Geometry check sheet. Reference: the model listing, model coordinates, mm. Face numbers are marked on the shaded views. A direction names the side the tool comes from. Round coordinates to 2 decimals unless told otherwise and drop trailing zeros. Write each loop counter-clockwise with the first axis right and the second up, starting at its lowest first coordinate (ties: lowest second). Pieces come first, ordered by that corner, then holes. Notation, with made-up numbers: (29, -15) -> (50, -15) arc R9 ccw to (50, -1) -> close; hole circle Ø8 at (47.5, 32). An arc over 180 degrees is marked (long way). One line per question, with ' | ' between items.
Autodesk Inventor part; units mm, degrees
ref_plane "YZ Plane" through (0, 0, 0) normal (1, 0, 0) x (0, 1, 0)
ref_plane "XZ Plane" through (0, 0, 0) normal (0, 1, 0) x (-1, 0, 0)
ref_plane "XY Plane" through (0, 0, 0) normal (0, 0, 1) x (1, 0, 0)
sketch "スケッチ1" plane through (0, 0, 0) normal (0, 0, 1) x (1, 0, 0)
  arc A0 (-1.55, 2.6268) -> (1.55, 2.6268) centre (0, 0) ccw
  circle A1 centre (-7, 0) radius 1.6
  circle A2 centre (7, 0) radius 1.6
  arc A3 (-7, 4) -> (-11, 0) centre (-7, 0) ccw
  arc A4 (11, 0) -> (7, 4) centre (7, 0) ccw
  line L0 (-1.55, 10) -> (-1.55, 2.6268)
  line L1 (1.55, 10) -> (1.55, 2.6268)
  circle A5 centre (0, -7) radius 1.6
  line L2 (1.55, 10) -> (5.55, 10)
  line L3 (5.55, 10) -> (5.55, 7.5385)
  line L4 (5.55, 4) -> (7, 4)
  line L5 (-1.55, 10) -> (-5.55, 10)
  line L6 (-5.55, 10) -> (-5.55, 7.5385)
  line L7 (-5.55, 4) -> (-7, 4)
  line L8 (-11, 0) -> (-11, -3)
  arc A6 (-11, -3) -> (-6.7837, -5.7424) centre (-8, -3) ccw
  arc A7 (1.55, 2.6268) -> (-1.55, 2.6268) centre (0, 0) ccw construction
  arc A8 (-3.9819, -7.3804) -> (3.9819, -7.3804) centre (0, -7) ccw
  arc A9 (-3.9819, -7.3804) -> (-6.7837, -5.7424) centre (-5.9728, -7.5706) ccw
  line L9 (11, 0) -> (11, -3)
  arc A10 (6.7837, -5.7424) -> (11, -3) centre (8, -3) ccw
  arc A11 (6.7837, -5.7424) -> (3.9819, -7.3804) centre (5.9728, -7.5706) ccw
  arc A12 (-5.55, 7.5385) -> (-5.55, 6.4615) centre (-6.95, 7) ccw construction
  arc A13 (5.55, 6.4615) -> (5.55, 7.5385) centre (6.95, 7) ccw construction
  arc A14 (-5.55, 6.4615) -> (-5.55, 7.5385) centre (-6.95, 7) ccw
  arc A15 (5.55, 7.5385) -> (5.55, 6.4615) centre (6.95, 7) ccw
  line L10 (5.55, 6.4615) -> (5.55, 4)
  line L11 (5.55, 7.5385) -> (5.55, 6.4615) construction
  line L12 (-5.55, 6.4615) -> (-5.55, 4)
  line L13 (-5.55, 7.5385) -> (-5.55, 6.4615) construction
  dimension "d0" = 6.1
  dimension "d1" = 3.2
  dimension "d2" = 3.2
  dimension "d4" = 7
  dimension "d5" = 7
  dimension "d6" = 3.2
  dimension "d7" = 7
  dimension "d8" = 6
  dimension "d9" = 4
  dimension "d10" = 3.1
  dimension "d11" = 4
  dimension "d12" = 4
  dimension "d13" = 1.55
  dimension "d14" = 3
  dimension "d15" = 3
  dimension "d16" = 4
  dimension "d17" = 4
  dimension "d18" = 3
  dimension "d19" = 3
  dimension "d20" = 2
  dimension "d21" = 2
  dimension "d22" = 3
  dimension "d23" = 3
  dimension "d24" = 1.4
  dimension "d25" = 1.4
  dimension "d26" = 3
  dimension "d27" = 3
extrude "押し出し1" add sketch "スケッチ1" along normal blind 6
sketch "スケッチ2" plane through (5.55, 4, 0) normal (1, 0, 0) x (0, 0, -1)
  circle A0 centre (-3, 3) radius 1.6
  line L0 (0, 6) -> (-6, 6)
  point P0 (0, -4)
  dimension "d30" = 3.2
  dimension "d31" = 3
  dimension "d32" = 3
extrude "押し出し2" cut sketch "スケッチ2" against normal through all
fillet "フィレット1" radius 0.5 8 edges at (-5.55, 10, 3) (-1.55, 10, 3) (1.55, 10, 3) (5.55, 10, 3) (5.55, 4, 3) (-5.55, 4, 3) (-1.55, 2.6268, 3) (1.55, 2.6268, 3)
properties part number "カップリング_軸6mm"
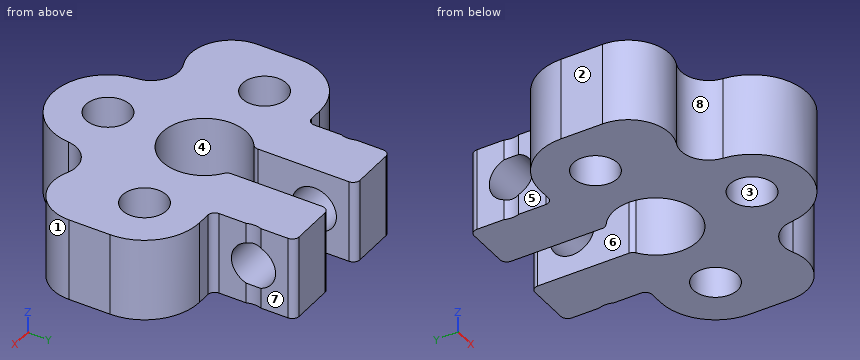
(1) Material ranges on line 1 (Y direction, x = 0, z = 4.6); line 2 (X direction, y = 1, z = 5.5); line 3 (X direction, y = -5.75, z = 1), recorded low to high.
Resolved:
line 1: y = -11 to -8.6, -5.4 to -3.05 | line 2: x = -10.87 to -8.25, -5.75 to -2.88, 2.88 to 5.75, 8.25 to 10.87 | line 3: x = -9.2 to -6.8, -5.14 to -1, 1 to 5.14, 6.8 to 9.2
(2) Sectioned sample at D-D on z = 4. Count the separate pieces of the cut face and the enclosed holes in it, then the cut area to 3 significant figures.
Resolved:
separate pieces: 3 | enclosed holes: 3 | area: 213 mm2
(3) Access from +Z, -Z, +X, -X, +Y, -Y to the whole of each face (thin tool, end or side, straight path). Record for the marked faces 4, 5, 6, 7 and 8.
Resolved:
face 4: +Z, -Z | face 5: +Z, -Z, -X, +Y | face 6: +Z, -Z, +Y | face 7: +Z, -Z, +X, +Y | face 8: +Z, -Z, -Y
(4) Sectioned sample at C-C on y = -7. Record the cut outline in (x, z).
Resolved:
outline: (-4.06, 0) -> (-1.6, 0) -> (-1.6, 6) -> (-4.06, 6) -> close; (1.6, 0) -> (4.06, 0) -> (4.06, 6) -> (1.6, 6) -> close
(5) Sectioned sample at A-A on x = 0. Record the cut outline in (y, z), then the cut area to 3 significant figures.
Resolved:
outline: (-11, 0) -> (-8.6, 0) -> (-8.6, 6) -> (-11, 6) -> close; (-5.4, 0) -> (-3.05, 0) -> (-3.05, 6) -> (-5.4, 6) -> close | area: 28.5 mm2
(6) Draft check along Y on the marked faces 1, 2 and 3. Enter one of: +Y half, -Y half, draft (parallel to the pull), parting line (faces both ways), or undercut.
Resolved:
face 1: -Y half | face 2: draft | face 3: undercut
(7) Sectioned sample at B-B on y = 7. Record the cut outline in (x, z), then the cut area to 3 significant figures.
Resolved:
outline: (-5.45, 0) -> (-1.55, 0) -> (-1.55, 1.4) -> (-5.45, 1.4) -> close; (-5.45, 4.6) -> (-1.55, 4.6) -> (-1.55, 6) -> (-5.45, 6) -> close; (1.55, 0) -> (5.45, 0) -> (5.45, 1.4) -> (1.55, 1.4) -> close; (1.55, 4.6) -> (5.45, 4.6) -> (5.45, 6) -> (1.55, 6) -> close | area: 21.8 mm2
(8) Go/stop test with flat-tipped pins: pin 1 (1.9 mm diameter, centred on y = 7, z = 3, fed in from -X); pin 2 (1 mm diameter, centred on y = 8, z = 4, fed in from +X); pin 3 (1 mm diameter, centred on x = -6.5, z = 4, fed in from +Y); pin 4 (0.6 mm diameter, centred on y = 5.5, z = 4, fed in from -X). Record where each tip stops, or that it passes through.
Resolved:
pin 1: passes through | pin 2: stops at x = 5.55 | pin 3: stops at y = 4 | pin 4: stops at x = -5.55
